```python
from build123d import *

# Parameters (mm, degrees)
F0_R     = 3.175
F1_DEPTH = 3.048


with BuildPart() as f1:
    # F0 (on Front) → F1 (new body)
    with BuildSketch(Plane.XZ):
        with BuildLine():
            ThreePointArc((-16.9247666998, 21.4792444312), (-22.070918521, 11.293529333), (-32.7201922638, 7.1917444312))
            Line((-32.7201922638, 7.1917444312), (-32.7201922638, -30.9082555688))
            ThreePointArc((-32.7201922638, -30.9082555688), (-25.985000173, -33.698063478), (-23.1951922638, -40.4332555688))
            Line((-23.1951922638, -40.4332555688), (3.7923077362, -40.4332555688))
            ThreePointArc((3.7923077362, -40.4332555688), (6.2182849547, -34.7212486641), (12.013289879, -32.5008193651))
            Line((12.013289879, -32.5008193651), (-13.7525922633, -31.5800218579))
            ThreePointArc((-13.7525922633, -31.5800218579), (-19.4589923665, -28.8618964189), (-21.3790056715, -22.8398737564))
            Line((-21.3790056715, -22.8398737564), (-16.9247666998, 21.4792444312))
        make_face()
        with BuildLine():
            ThreePointArc((-32.7201922638, 7.1917444312), (-42.0272444513, 10.2061688384), (-47.7997573919, 18.1046540905))
            Line((-47.7997573919, 18.1046540905), (-42.2032386499, -41.326259622))
            ThreePointArc((-42.2032386499, -41.326259622), (-39.7640366902, -34.0215568316), (-32.7201922638, -30.9082555688))
            Line((-32.7201922638, -30.9082555688), (-32.7201922638, 7.1917444312))
        make_face()
        with BuildLine():
            ThreePointArc((-23.1951922638, 73.8667444312), (-25.985000173, 67.1315523404), (-32.7201922638, 64.3417444312))
            Line((-32.7201922638, 64.3417444312), (-32.7201922638, 59.5919444312))
            Line((-32.7201922638, 59.5919444312), (-32.7201922638, 38.9417444312))
            ThreePointArc((-32.7201922638, 38.9417444312), (-22.2201134041, 34.9732119568), (-16.9697862216, 25.051772014))
            Line((-16.9697862216, 25.051772014), (-23.2470820733, 74.8596232349))
            ThreePointArc((-23.2470820733, 74.8596232349), (-23.2081735621, 74.3638613368), (-23.1951922638, 73.8667444312))
        make_face()
        with BuildLine():
            ThreePointArc((-16.9697862216, 25.051772014), (-22.2201134041, 34.9732119568), (-32.7201922638, 38.9417444312))
            Line((-32.7201922638, 38.9417444312), (-32.7201922638, 26.2417444312))
            ThreePointArc((-32.7201922638, 26.2417444312), (-30.4751282336, 25.3118084615), (-29.5451922638, 23.0667444312))
            ThreePointArc((-29.5451922638, 23.0667444312), (-30.4751282336, 20.821680401), (-32.7201922638, 19.8917444312))
            Line((-32.7201922638, 19.8917444312), (-32.7201922638, 7.1917444312))
            ThreePointArc((-32.7201922638, 7.1917444312), (-22.070918521, 11.293529333), (-16.9247666998, 21.4792444312))
            ThreePointArc((-16.9247666998, 21.4792444312), (-16.8650983532, 22.2719978772), (-16.8451922638, 23.0667444312))
            ThreePointArc((-16.8451922638, 23.0667444312), (-16.8763713718, 24.0612113938), (-16.9697862216, 25.051772014))
        make_face()
        with BuildLine():
            Line((-32.7201922638, 26.2417444312), (-32.7201922638, 38.9417444312))
            ThreePointArc((-32.7201922638, 38.9417444312), (-43.1919774337, 34.9981039664), (-48.4609965266, 25.1265274684))
            Line((-48.4609965266, 25.1265274684), (-47.7997573919, 18.1046540905))
            ThreePointArc((-47.7997573919, 18.1046540905), (-42.0272444513, 10.2061688384), (-32.7201922638, 7.1917444312))
            Line((-32.7201922638, 7.1917444312), (-32.7201922638, 19.8917444312))
            ThreePointArc((-32.7201922638, 19.8917444312), (-35.8951922638, 23.0667444312), (-32.7201922638, 26.2417444312))
        make_face()
        with BuildLine():
            Line((-32.7201922638, 59.5919444312), (-32.7201922638, 64.3417444312))
            ThreePointArc((-32.7201922638, 64.3417444312), (-39.1263785452, 66.8178862025), (-42.2018298248, 72.9589040472))
            Line((-42.2018298248, 72.9589040472), (-48.4609965266, 25.1265274684))
            ThreePointArc((-48.4609965266, 25.1265274684), (-43.1919774337, 34.9981039664), (-32.7201922638, 38.9417444312))
            Line((-32.7201922638, 38.9417444312), (-32.7201922638, 59.5919444312))
        make_face()
        with Locations((-35.8951922638, 59.5919444312)):
            Circle(F0_R, mode=Mode.SUBTRACT)
        with BuildLine():
            ThreePointArc((-42.2018298248, 72.9589040472), (-39.1263785452, 66.8178862025), (-32.7201922638, 64.3417444312))
            ThreePointArc((-32.7201922638, 64.3417444312), (-25.985000173, 67.1315523404), (-23.1951922638, 73.8667444312))
            ThreePointArc((-23.1951922638, 73.8667444312), (-23.2081735621, 74.3638613368), (-23.2470820733, 74.8596232349))
            ThreePointArc((-23.2470820733, 74.8596232349), (-31.5267060991, 83.3166764826), (-41.6489880278, 77.1837055714))
            Line((-41.6489880278, 77.1837055714), (-42.2018298248, 72.9589040472))
        make_face()
        with BuildLine():
            ThreePointArc((-29.5451922638, 73.8667444312), (-30.4751282336, 71.621680401), (-32.7201922638, 70.6917444312))
            ThreePointArc((-32.7201922638, 70.6917444312), (-34.9652562941, 76.1118084615), (-29.5451922638, 73.8667444312))
        make_face(mode=Mode.SUBTRACT)
        with BuildLine():
            ThreePointArc((-23.1951922638, -40.4332555688), (-25.8657839782, -47.0470829065), (-32.3800136924, -49.9521790131))
            Line((-32.3800136924, -49.9521790131), (12.013289879, -48.3656917724))
            ThreePointArc((12.013289879, -48.3656917724), (6.2182849547, -46.1452624735), (3.7923077362, -40.4332555688))
            Line((3.7923077362, -40.4332555688), (-23.1951922638, -40.4332555688))
        make_face()
        with BuildLine():
            ThreePointArc((3.7923077362, -40.4332555688), (6.2182849547, -46.1452624735), (12.013289879, -48.3656917724))
            ThreePointArc((12.013289879, -48.3656917724), (17.4418146409, -45.9447783502), (19.6673077362, -40.4332555688))
            ThreePointArc((19.6673077362, -40.4332555688), (17.4418146409, -34.9217327873), (12.013289879, -32.5008193651))
            ThreePointArc((12.013289879, -32.5008193651), (6.2182849547, -34.7212486641), (3.7923077362, -40.4332555688))
        make_face()
        with BuildLine():
            ThreePointArc((14.9048077362, -40.4332555688), (11.7298077362, -43.6082555688), (8.5548077362, -40.4332555688))
            ThreePointArc((8.5548077362, -40.4332555688), (11.7298077362, -37.2582555688), (14.9048077362, -40.4332555688))
        make_face(mode=Mode.SUBTRACT)
        with BuildLine():
            ThreePointArc((-32.7201922638, -30.9082555688), (-39.7640366902, -34.0215568316), (-42.2032386499, -41.326259622))
            ThreePointArc((-42.2032386499, -41.326259622), (-39.0050653178, -47.5904893707), (-32.3800136924, -49.9521790131))
            ThreePointArc((-32.3800136924, -49.9521790131), (-25.8657839782, -47.0470829065), (-23.1951922638, -40.4332555688))
            Line((-23.1951922638, -40.4332555688), (-29.5451922638, -40.4332555688))
            ThreePointArc((-29.5451922638, -40.4332555688), (-34.9652562941, -42.678319599), (-32.7201922638, -37.2582555688))
            Line((-32.7201922638, -37.2582555688), (-32.7201922638, -30.9082555688))
        make_face()
        with BuildLine():
            ThreePointArc((-23.1951922638, -40.4332555688), (-25.985000173, -33.698063478), (-32.7201922638, -30.9082555688))
            Line((-32.7201922638, -30.9082555688), (-32.7201922638, -37.2582555688))
            ThreePointArc((-32.7201922638, -37.2582555688), (-30.4751282336, -38.1881915385), (-29.5451922638, -40.4332555688))
            Line((-29.5451922638, -40.4332555688), (-23.1951922638, -40.4332555688))
        make_face()
        with Locations((-35.8951922638, 59.5919444312)):
            Circle(F0_R)
        with BuildLine():
            ThreePointArc((-29.5451922638, 73.8667444312), (-34.9652562941, 76.1118084615), (-32.7201922638, 70.6917444312))
            ThreePointArc((-32.7201922638, 70.6917444312), (-30.4751282336, 71.621680401), (-29.5451922638, 73.8667444312))
        make_face()
        with BuildLine():
            ThreePointArc((14.9048077362, -40.4332555688), (11.7298077362, -37.2582555688), (8.5548077362, -40.4332555688))
            ThreePointArc((8.5548077362, -40.4332555688), (11.7298077362, -43.6082555688), (14.9048077362, -40.4332555688))
        make_face()
        with BuildLine():
            Line((-32.7201922638, -40.4332555688), (-32.7201922638, -37.2582555688))
            ThreePointArc((-32.7201922638, -37.2582555688), (-34.9652562941, -42.678319599), (-29.5451922638, -40.4332555688))
            Line((-29.5451922638, -40.4332555688), (-32.7201922638, -40.4332555688))
        make_face()
        with BuildLine():
            ThreePointArc((-29.5451922638, 23.0667444312), (-30.4751282336, 25.3118084615), (-32.7201922638, 26.2417444312))
            Line((-32.7201922638, 26.2417444312), (-32.7201922638, 19.8917444312))
            ThreePointArc((-32.7201922638, 19.8917444312), (-30.4751282336, 20.821680401), (-29.5451922638, 23.0667444312))
        make_face()
        with BuildLine():
            Line((-32.7201922638, 19.8917444312), (-32.7201922638, 26.2417444312))
            ThreePointArc((-32.7201922638, 26.2417444312), (-35.8951922638, 23.0667444312), (-32.7201922638, 19.8917444312))
        make_face()
        with BuildLine():
            ThreePointArc((-29.5451922638, -40.4332555688), (-30.4751282336, -38.1881915385), (-32.7201922638, -37.2582555688))
            Line((-32.7201922638, -37.2582555688), (-32.7201922638, -40.4332555688))
            Line((-32.7201922638, -40.4332555688), (-29.5451922638, -40.4332555688))
        make_face()
        with BuildLine():
            Line((-47.7997573919, 18.1046540905), (-48.4609965266, 25.1265274684))
            ThreePointArc((-48.4609965266, 25.1265274684), (-48.525269574, 21.5784043426), (-47.7997573919, 18.1046540905))
        make_face()
        with BuildLine():
            ThreePointArc((-41.6489880278, 77.1837055714), (-42.1646748215, 75.1026142535), (-42.2018298248, 72.9589040472))
            Line((-42.2018298248, 72.9589040472), (-41.6489880278, 77.1837055714))
        make_face()
    extrude(amount=F1_DEPTH)


solid = f1.part
```
Geometry check sheet. Reference: the model listing, model coordinates, mm. Coordinates: 2 decimals unless noted, no trailing zeros. Write each loop counter-clockwise with the first axis right and the second up, starting at its lowest first coordinate (ties: lowest second). Pieces come first, ordered by that corner, then holes. Notation, with made-up numbers: M 8,-26.5 L 45,-26.5 A25 ccw 45,-13.5 Z; hole C 46.25,60 d11. An arc over 180 degrees is marked long. Use one line per item in the form item = value. Start each with the question number.
1) Release check for a two-part mould opening along Z. For faces 1 (the cylindrical face through (-48.53, -1.5, 21.63)), 2 (the flat face through (-45.04, -1.5, -11.19)), 3 (the flat face through (-20.064, -1.503, 49.607)), 4 (the flat face through (-19.183, -1.503, -0.991)) record: pulls with the +Z half, pulls with the -Z half, needs draft (parallel to the pull), parting line crosses it, or undercut.
2) Thickness scan on probe 1 along X at (y, z) = (-0.35, 36.5); probe 2 along Z at (x, y) = (-37, -1.7); probe 3 along Z at (x, y) = (-7.5, -2.45). Record the ranges inside material, lowest first. Write a range as from..to.
3) Go/stop test with flat-tipped pins: pin 1 Ø1 at (y, z) = (-0.5, 40) entering from +X; pin 2 Ø1 at (y, z) = (-2.5, 70) entering from -X. Record where each tip stops, or that it passes through.
4) Section check B-B on z = 50. Enter the section's corners in (x, y), and give its area (3 significant figures).
5) Section check C-C on x = 14. Enter the section's corners in (y, z).
Responses:
q1.face_1 = parting line crosses it
q1.face_2 = pulls with the -Z half
q1.face_3 = pulls with the +Z half
q1.face_4 = undercut
q2.probe_1 = -46.97..-18.41
q2.probe_2 = -48.94..82.38
q2.probe_3 = -49.06..-31.8
q3.pin_1 = -18.79
q3.pin_2 = -42.65
q4.outline = M -45.21,-3.05 L -20.11,-3.05 L -20.11,0 L -45.21,0 Z
q4.area = 76.5 mm2
q5.outline = M -3.05,-48.04 L 0,-48.04 L 0,-32.83 L -3.05,-32.83 Z
